```python
from build123d import *

# Parameters (mm, degrees)
SKETCH1_R           = 0.5
BOSS_EXTRUDE1_DEPTH = 2
FILLET1_R           = 5


with BuildPart() as part:
    # Sketch1 → Boss-Extrude1 (new body)
    with BuildSketch(Plane.XY):
        with BuildLine():
            Line((0, 0), (3.3, 0))
            ThreePointArc((3.3, 0), (5, 1.7), (6.7, 0))
            Line((6.7, 0), (10, 0))
            ThreePointArc((10, 0), (11.7, -1.7), (10, -3.4))
            Line((10, -3.4), (6.7, -3.4))
            ThreePointArc((6.7, -3.4), (5, -5.1), (3.3, -3.4))
            Line((3.3, -3.4), (-0.1, -3.4))
            ThreePointArc((-0.1, -3.4), (-1.800735135, -1.64850779), (0, 0))
        make_face()
        with Locations((-0.1, -1.698529412)):
            Circle(SKETCH1_R, mode=Mode.SUBTRACT)
        with Locations((10, -1.7)):
            Circle(SKETCH1_R, mode=Mode.SUBTRACT)
        with Locations((5, -1.7)):
            Circle(SKETCH1_R, mode=Mode.SUBTRACT)
    extrude(amount=BOSS_EXTRUDE1_DEPTH)

    # Fillet1
    fillet1_edges = [part.edges().sort_by_distance(p)[0] for p in [
        (3.3, 0, 1),
        (6.7, 0, 1),
        (6.7, -3.4, 1),
        (3.3, -3.4, 1),
    ]]
    fillet(fillet1_edges, radius=FILLET1_R)


solid = part.part
```
Geometry: final body of the model. Coordinates: model frame, mm. Coordinates: 2 decimals unless noted, no trailing zeros. Order: outer loops, then holes, each group sorted by start corner. A loop starts at its lowest first (then second) coordinate and runs counter-clockwise, first axis right, second up. Notation, with made-up numbers: M 34,-18.75 L 88,-18.75 A18 ccw 88,16.25 Z; hole C -19.75,-12 d11. An arc over 180 degrees is marked long. Answer in a Markdown table with one row per item. Add a question column.
Q1. Section query C-C on z = 0.3. Return the cut outline in (x, y), and give its area (3 significant figures).
Q2. Line query: L1, parallel to Y at x = -0.1, z = 1.5; L2, parallel to Y at x = 5, z = 0.55; L3, parallel to Y at x = 1.5, z = 0.1. Output: solid intervals per line, ascending.
Q3. Section query A-A on x = 5. Return the cut outline in (y, z).
Q4. Section query B-B on y = -2. Return the cut outline in (x, z).
Q5. Mould query, pull axis Y, two halves, no side actions, for faces 1 (the cylindrical face through (0.2, -1.3, 1)), 2 (the cylindrical face through (2.3, 0.32, 1.01)), 3 (the flat face through (5, -2.4, 2)). Classes: released by +Y, released by -Y, zero draft, split by the parting line, or undercut.
Q6. Section query D-D on x = 10.25. Return the cut outline in (y, z).
Completed:
| question | item | result |
|---|---|---|
| 1 | outline | M -0.1,-3.4 L 0.54,-3.4 A5 cw 3.87,-4.67 A1.7 ccw 6.13,-4.67 A5 cw 9.46,-3.4 L 10,-3.4 A1.7 ccw 10,0 L 9.46,0 A5 cw 6.13,1.27 A1.7 ccw 3.87,1.27 A5 cw 0.54,0 L 0,0 A1.7 ccw long Z; hole C -0.1,-1.7 d1; hole C 5,-1.7 d1; hole C 10,-1.7 d1 |
| 1 | area | 53.5 mm2 |
| 2 | L1 | y = -3.4 to -2.2, -1.2 to 0 |
| 2 | L2 | y = -5.1 to -2.2, -1.2 to 1.7 |
| 2 | L3 | y = -3.49 to 0.09 |
| 3 | outline | M -5.1,0 L -2.2,0 L -2.2,2 L -5.1,2 Z; M -1.2,0 L 1.7,0 L 1.7,2 L -1.2,2 Z |
| 4 | outline | M -1.77,0 L -0.5,0 L -0.5,2 L -1.77,2 Z; M 0.3,0 L 4.6,0 L 4.6,2 L 0.3,2 Z; M 5.4,0 L 9.6,0 L 9.6,2 L 5.4,2 Z; M 10.4,0 L 11.67,0 L 11.67,2 L 10.4,2 Z |
| 5 | face 1 | undercut |
| 5 | face 2 | released by +Y |
| 5 | face 3 | zero draft |
| 6 | outline | M -3.38,0 L -2.13,0 L -2.13,2 L -3.38,2 Z; M -1.27,0 L -0.02,0 L -0.02,2 L -1.27,2 Z |
